Autodesk Inventor part; units mm, degrees
ref_plane "Work Plane1" through (0, -37.5, 0) normal (-1, 0, 0) x (0, 0, 1)
ref_plane "YZ Plane" through (0, 0, 0) normal (1, 0, 0) x (0, 1, 0)
ref_plane "XZ Plane" through (0, 0, 0) normal (0, 1, 0) x (-1, 0, 0)
sketch "Sketch1" plane through (0, 0, 0) normal (0, 0, 1) x (1, 0, 0)
  line L0 (-12.5, 12.5) -> (12.5, 12.5)
  line L1 (12.5, 12.5) -> (12.5, -37.5)
  line L2 (12.5, -37.5) -> (-12.5, -37.5)
  line L3 (-12.5, -37.5) -> (-12.5, 12.5)
  point P0 (0, 0)
  dimension "d0" = 25
  dimension "d1" = 50
  dimension "d2" = 12.5
  dimension "d3" = 12.5
extrude "Extrusion1" add sketch "Sketch1" along normal blind 10
sketch "Sketch2" plane through (0, 0, 0) normal (0, 0, -1) x (-1, 0, 0)
  circle A0 centre (0, -33) radius 1.5
  circle A1 centre (0, 0) radius 7.5
  dimension "d7" = 3
  dimension "d8" = 33
  dimension "d17" = 15
extrude "Extrusion2" add sketch "Sketch2" along normal blind 6 contours A0
sketch "Sketch3" plane through (0, 0, 10) normal (0, 0, 1) x (1, 0, 0)
  arc A0 (7.5, 0) -> (-7.5, 0) centre (0, 0) ccw
  line L0 (-7.5, 0) -> (-12.5, 0)
  line L1 (-12.5, 12.5) -> (-12.5, -37.5)
  line L2 (-12.5, 0) -> (-12.5, 12.5)
  line L3 (12.5, 12.5) -> (-12.5, 12.5)
  line L4 (12.5, 12.5) -> (12.5, 0)
  line L5 (12.5, -37.5) -> (12.5, 12.5)
  line L6 (7.5, 0) -> (12.5, 0)
  dimension "d11" = 15
extrude "Extrusion3" add sketch "Sketch3" along normal blind 15
sketch "Sketch4" plane through (0, 0, 25) normal (0, 0, 1) x (1, 0, 0)
  line L0 (-12.5, 12.5) -> (-12.5, 0)
  line L1 (-12.5, 12.5) -> (12.5, 12.5)
  line L2 (12.5, 12.5) -> (12.5, -17.5)
  line L3 (12.5, -17.5) -> (-12.5, -17.5)
  line L4 (-12.5, -17.5) -> (-12.5, 12.5)
  point P0 (0, 0)
  dimension "d14" = 25
  dimension "d21" = 30
extrude "Extrusion4" add sketch "Sketch4" along normal blind 10
sketch "Sketch5" plane through (0, 0, 0) normal (0, 0, -1) x (-1, 0, 0)
  circle A0 centre (0, 0) radius 7.5
  dimension "d18" = 15
extrude "Extrusion5" cut sketch "Sketch5" against normal blind 10
sketch "Sketch6" plane through (0, 0, 10) normal (0, 0, 1) x (1, 0, 0)
  line L0 (-12.5, -20.5) -> (-12.5, -37.5)
  line L1 (-12.5, -37.5) -> (12.5, -37.5)
  line L2 (-12.5, -37.5) -> (12.5, -37.5)
  line L3 (12.5, -37.5) -> (12.5, -20.5)
  line L4 (12.5, -37.5) -> (12.5, 0)
  arc A0 (-7.5, -20.5) -> (7.5, -20.5) centre (0, -20.5) ccw
  line L5 (-12.5, -20.5) -> (-7.5, -20.5)
  line L6 (7.5, -20.5) -> (12.5, -20.5)
  line L7 (-12.5, 0) -> (-12.5, -37.5)
  line L8 (-12.5, -29) -> (12.5, -29)
  point P0 (0, 0)
  dimension "d22" = 15
  dimension "d23" = 17
  dimension "d24" = 17
ref_plane "Work Plane1" through (0, -37.5, 0) normal (-1, 0, 0) x (0, 0, 1)
sketch "Sketch8" plane through (0, -37.5, 0) normal (-1, 0, 0) x (0, 0, 1)
  line L0 (10, 0) -> (10, 37.5)
  line L1 (10, 8.5) -> (35, -0.5993)
  line L2 (10, 8.5) -> (36.6044, 8.5) construction
  line L3 (0, 0) -> (10, 0)
  point P0 (0, 37.5)
  dimension "d26" = 20
  dimension "d27" = 8.5
  dimension "d32" = 25
sweep "Sweep1" add profiles "Sketch6" path "Sketch8" path curves L1
thread "Thread1"
equation "\"d24\" = d23"
properties part number "top_part"
Check sheet for the modelled part. Datum: model origin and axes. Units: mm. A direction names the side the tool comes from. Coordinates: 2 decimals unless noted, no trailing zeros. Order: outer loops, then holes, each group sorted by start corner. A loop starts at its lowest first (then second) coordinate and runs counter-clockwise, first axis right, second up. Notation, with made-up numbers: (81.25, 55.5) -> (112.25, 55.5) arc R29 ccw to (112.25, 85.5) -> close; hole circle Ø6 at (66, -13.75). An arc over 180 degrees is marked (long way). Write each question's results on one line, items separated by ' | '. Start each with the question number.
1) Draft check along X on faces 5 (the face through (-0.494, 7.484, 9.547)), 6 (the face through (0, -40, 35)), 7 (the face through (0.325, -31.536, -2.958)). Enter one of: pulls with the +X half, pulls with the -X half, needs draft (parallel to the pull), parting line crosses it, or undercut.
2) Depth check by flat-ended pin: pin 1 (3 mm diameter, centred on x = -3.5, z = 6, fed in from -Y); pin 2 (7.5 mm diameter, centred on x = -2, y = -18, fed in from -Z); pin 3 (9 mm diameter, centred on x = 0, y = 0, fed in from -Z). Enter the tip coordinate at first touch or a pass-through.
3) Set-up check for faces 1 (the face through (-10, 0, 17)), 2 (the face through (0, -17.5, 30)), 3 (the face through (0, -37.5, 5)), 4 (the face through (0, -8, 25)): record each of +Z, -Z, +X, -X, +Y, -Y from which the full face is reachable in a straight line by a thin tool's end or side.
4) Section check C-C (x = 10.25). Enter the section's corners in (y, z).
5) Material ranges on line 1 along Z through (x, y) = (-0.5, -11); line 2 along X through (y, z) = (0, 6); line 3 along Z through (x, y) = (-1.5, 5), recorded low to high.
6) Section check B-B (z = 7). Enter the section's corners in (x, y).
7) Section check A-A (y = -11.5). Enter the section's corners in (x, z).
8) Section check D-D (y = -1). Enter the section's corners in (x, z).
Checked values:
1) face 5: undercut | face 6: needs draft | face 7: parting line crosses it
2) pin 1: y = -37.5 | pin 2: z = 0 | pin 3: z = 25
3) face 1: +X, -X | face 2: +Z, +X, -X | face 3: -Z, +X, -X, -Y | face 4: none
4) outline: (-46.6, 35) -> (-37.5, 10) -> (-37.5, 0) -> (12.5, 0) -> (12.5, 35) -> (-17.5, 35) -> (-17.5, 25) -> (0, 25) -> (0, 10) -> (-20.5, 10) -> (-29.6, 35) -> close
5) line 1: 0 to 10, 25 to 35 | line 2: -12.5 to -7.5, 7.5 to 12.5 | line 3: 25 to 35
6) outline: (-12.5, -37.5) -> (12.5, -37.5) -> (12.5, 12.5) -> (-12.5, 12.5) -> close; hole circle Ø15 at (0, 0)
7) outline: (-12.5, 0) -> (12.5, 0) -> (12.5, 10) -> (-12.5, 10) -> close; (-12.5, 25) -> (12.5, 25) -> (12.5, 35) -> (-12.5, 35) -> close
8) outline: (-12.5, 0) -> (-7.43, 0) -> (-7.43, 10) -> (-12.5, 10) -> close; (-12.5, 25) -> (12.5, 25) -> (12.5, 35) -> (-12.5, 35) -> close; (7.43, 0) -> (12.5, 0) -> (12.5, 10) -> (7.43, 10) -> close
